The listing builds one solid part. Answer for the finished solid, in the listing's coordinates (mm). Face numbers are marked on the shaded views. Coordinates: 2 decimals unless noted, no trailing zeros. Loops run counter-clockwise (first coordinate to the right, second up) from the corner with the lowest first, then second, coordinate; pieces in that order, holes last. Notation, with made-up numbers: (42.5, 33.5) - (70.5, 33.5) arc R22 cw to (70.5, 48.5) - close; hole circle Ø3 at (87, 6). An arc over 180 degrees is marked (long way). Return JSON: item names as keys, results as strings. Group by question number.
1. Section B-B (x = 45) is taken. Write down the section's boundary in (y, z), and give its area (3 significant figures).
2. Section D-D (z = 45) is taken. Write down the section's boundary in (x, y).
3. Find the intervals of material crossed by line 1 along X through (y, z) = (88.4, 0); line 2 along Y through (x, z) = (-25.5, -54), in increasing order.
4. Section A-A (z = 0) is taken. Write down the section's boundary in (x, y).
5. The mould has two halves that part along Y. Classify the marked faces 1, 2 and 3: pulls with the +Y half, pulls with the -Y half, needs draft (parallel to the pull), parting line crosses it, or undercut.
6. Each of these flat-tipped pins is pushed along its axis until it touches: P1, Ø12, axis at x = -46.5, y = 26, coming from the -Z side; P2, Ø4, axis at x = -40.5, y = 61, coming from the -Z side; P3, Ø12, axis at x = 0, z = 0, coming from the +Y side. Where does it stop, or does it pass through?
7. Section C-C (x = -15) is taken. Write down the section's boundary in (y, z).
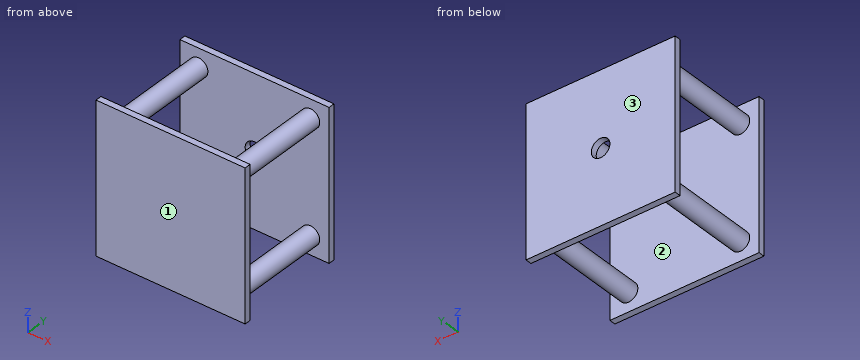
Autodesk Inventor part; units mm, degrees
ref_plane "YZ Plane" through (0, 0, 0) normal (1, 0, 0) x (0, 1, 0)
ref_plane "XZ Plane" through (0, 0, 0) normal (0, 1, 0) x (-1, 0, 0)
ref_plane "XY Plane" through (0, 0, 0) normal (0, 0, 1) x (1, 0, 0)
sketch "Boceto1" plane through (0, 0, 0) normal (0, 1, 0) x (-1, 0, 0)
  line L0 (60, -60) -> (-60, -60)
  line L1 (-60, -60) -> (-60, 60)
  line L2 (-60, 60) -> (60, 60)
  line L3 (60, 60) -> (60, -60)
  line L4 (60, -60) -> (-60, 60) construction
  line L5 (-60, -60) -> (60, 60) construction
  point P0 (0, 0)
  dimension "d0" = 120
  dimension "d1" = 120
extrude "Extrusión1" add sketch "Boceto1" along normal blind 5
sketch "Boceto2" plane through (0, 5, 0) normal (0, 1, 0) x (1, 0, 0)
  line L0 (45, -45) -> (-45, -45)
  line L1 (-45, -45) -> (-45, 45)
  line L2 (-45, 45) -> (45, 45)
  line L3 (45, 45) -> (45, -45)
  line L4 (45, -45) -> (-45, 45) construction
  line L5 (-45, -45) -> (45, 45) construction
  circle A0 centre (-45, 45) radius 7.5
  circle A1 centre (45, 45) radius 7.5
  circle A2 centre (-45, -45) radius 7.5
  circle A3 centre (45, -45) radius 7.5
  point P0 (0, 0)
  dimension "d4" = 90
  dimension "d5" = 90
  dimension "d6" = 15
  dimension "d7" = 15
  dimension "d8" = 15
  dimension "d9" = 15
extrude "Extrusión2" add sketch "Boceto2" along normal blind 80 contours A2 L1 L0 | L0 L1 A2 | A3 L3 L0 | L0 L3 A3 | A0 L2 L1 | L1 L2 A0 | A1 L2 L3 | L3 L2 A1
sketch "Boceto3" plane through (-45, 85, 45) normal (0, 1, 0) x (1, 0, 0)
  circle A0 centre (90, 90) radius 7.5
  line L0 (90, 90) -> (-30, 90)
  line L1 (-30, 90) -> (-30, -30)
  line L2 (-30, -30) -> (90, -30)
  line L3 (90, -30) -> (90, 90)
  line L4 (-15, 105) -> (105, 105)
  line L5 (105, 105) -> (105, -15)
  line L6 (105, -15) -> (-15, -15)
  line L7 (-15, -15) -> (-15, 105)
  line L8 (-15, 105) -> (105, -15) construction
  line L9 (105, 105) -> (-15, -15) construction
  point P0 (45, 45)
  dimension "d12" = 120
  dimension "d13" = 120
extrude "Extrusión3" add sketch "Boceto3" along normal blind 5 contours A0 L3 L0 | A0 L0 L7 L4 L5 L6 L3 | L0 L3 A0 | A0 L3 L6 L7 L0
sketch "Boceto4" plane through (-45, 90, 45) normal (0, 1, 0) x (1, 0, 0)
  circle A0 centre (45, 45) radius 7.5
  dimension "d16" = 15
extrude "Extrusión4" cut sketch "Boceto4" against normal blind 10
properties part number "Central_base" material "Plástico ABS"
The answers:
{
 "1": {"outline": "(0, -60) - (5, -60) - (5, -52.5) - (85, -52.5) - (85, -60) - (90, -60) - (90, 60) - (85, 60) - (85, 52.5) - (5, 52.5) - (5, 60) - (0, 60) - close; hole (5, -37.5) - (85, -37.5) - (85, 37.5) - (5, 37.5) - close", "area": "3,600 mm2"},
 "2": {"outline": "(-60, 0) - (60, 0) - (60, 5) - (52.5, 5) - (52.5, 85) - (60, 85) - (60, 90) - (-60, 90) - (-60, 85) - (-52.5, 85) - (-52.5, 5) - (-60, 5) - close; hole (-37.5, 5) - (37.5, 5) - (37.5, 85) - (-37.5, 85) - close"},
 "3": {"line 1": "x = -60 to -7.5, 7.5 to 60", "line 2": "y = 0 to 5, 85 to 90"},
 "4": {"outline": "(-60, 0) - (60, 0) - (60, 5) - (-60, 5) - close; (-60, 85) - (-7.5, 85) - (-7.5, 90) - (-60, 90) - close; (7.5, 85) - (60, 85) - (60, 90) - (7.5, 90) - close"},
 "5": {"face 1": "pulls with the -Y half", "face 2": "undercut", "face 3": "pulls with the +Y half"},
 "6": {"P1": "stops at z = -52.5", "P2": "stops at z = -52.07", "P3": "stops at y = 5"},
 "7": {"outline": "(0, -60) - (5, -60) - (5, 60) - (0, 60) - close; (85, -60) - (90, -60) - (90, 60) - (85, 60) - close"}
}
